Here's how the part is built. I have some questions about the finished solid (model axes, mm). Round coordinates to 2 decimals unless told otherwise and drop trailing zeros. Loops run counter-clockwise (first coordinate to the right, second up) from the corner with the lowest first, then second, coordinate; pieces in that order, holes last. Notation, with made-up numbers: M 9,83.5 L 19,83.5 A17 ccw 19,102.5 Z; hole C -23.5,57 d6. An arc over 180 degrees is marked long. Answer as a JSON object with one key per item and string values.
from build123d import *

# Parameters (mm, degrees)
SKETCH1_W           = 250
SKETCH1_H           = 150
SKETCH1_R           = 1.5
SKETCH1_R_2         = 10
BOSS_EXTRUDE1_DEPTH = 4


with BuildPart() as part:
    # Sketch1 → Boss-Extrude1 (new body)
    with BuildSketch(Plane.XY):
        with Locations((64.901502586, -41.133333333)):
            Rectangle(SKETCH1_W, SKETCH1_H)
        with Locations((-32.098497414, -92.133333333)):
            Circle(SKETCH1_R, mode=Mode.SUBTRACT)
        with Locations((-17.098497414, -92.133333333)):
            Circle(SKETCH1_R, mode=Mode.SUBTRACT)
        with Locations((-32.098497414, -107.133333333)):
            Circle(SKETCH1_R, mode=Mode.SUBTRACT)
        with Locations((-47.098497414, -92.133333333)):
            Circle(SKETCH1_R, mode=Mode.SUBTRACT)
        with Locations((-32.098497414, -77.133333333)):
            Circle(SKETCH1_R, mode=Mode.SUBTRACT)
        with Locations((176.901502586, -92.133333333)):
            Circle(SKETCH1_R, mode=Mode.SUBTRACT)
        with Locations((161.901502586, -92.133333333)):
            Circle(SKETCH1_R, mode=Mode.SUBTRACT)
        with Locations((161.901502586, -77.133333333)):
            Circle(SKETCH1_R, mode=Mode.SUBTRACT)
        with Locations((146.901502586, -92.133333333)):
            Circle(SKETCH1_R, mode=Mode.SUBTRACT)
        with Locations((161.901502586, -107.133333333)):
            Circle(SKETCH1_R, mode=Mode.SUBTRACT)
        with Locations((176.901502586, 9.866666667)):
            Circle(SKETCH1_R, mode=Mode.SUBTRACT)
        with Locations((161.901502586, 9.866666667)):
            Circle(SKETCH1_R, mode=Mode.SUBTRACT)
        with Locations((161.901502586, 24.866666667)):
            Circle(SKETCH1_R, mode=Mode.SUBTRACT)
        with Locations((146.901502586, 9.866666667)):
            Circle(SKETCH1_R, mode=Mode.SUBTRACT)
        with Locations((161.901502586, -5.133333333)):
            Circle(SKETCH1_R, mode=Mode.SUBTRACT)
        with Locations((-17.098497414, 9.866666667)):
            Circle(SKETCH1_R, mode=Mode.SUBTRACT)
        with Locations((-32.098497414, 9.866666667)):
            Circle(SKETCH1_R, mode=Mode.SUBTRACT)
        with Locations((-32.098497414, 24.866666667)):
            Circle(SKETCH1_R, mode=Mode.SUBTRACT)
        with Locations((-47.098497414, 9.866666667)):
            Circle(SKETCH1_R, mode=Mode.SUBTRACT)
        with Locations((-32.098497414, -5.133333333)):
            Circle(SKETCH1_R, mode=Mode.SUBTRACT)
        with Locations((-32.098497414, -41.133333333)):
            Circle(SKETCH1_R, mode=Mode.SUBTRACT)
        with Locations((161.901502586, -41.133333333)):
            Circle(SKETCH1_R, mode=Mode.SUBTRACT)
        with Locations((64.901502586, 9.866666667)):
            Circle(SKETCH1_R, mode=Mode.SUBTRACT)
        with Locations((64.901502586, -92.133333333)):
            Circle(SKETCH1_R, mode=Mode.SUBTRACT)
        with Locations((94.901502586, -41.133333333)):
            Circle(SKETCH1_R_2, mode=Mode.SUBTRACT)
        with Locations((34.901502586, -41.133333333)):
            Circle(SKETCH1_R_2, mode=Mode.SUBTRACT)
    extrude(amount=BOSS_EXTRUDE1_DEPTH)


solid = part.part
Item 1: If I drill on L1, parallel to X at y = 24.5, z = 2.3; L2, parallel to Y at x = 177.5, z = 0.65; L3, parallel to X at y = -76.5, z = 3.3, over which ranges is the centre line in solid material (lowest first)? Write a range as from..to.
Solution:
{"L1": "x = -60.1..-33.55, -30.64..160.45, 163.36..189.9", "L2": "y = -116.13..-93.51, -90.76..8.49, 11.24..33.87", "L3": "x = -60.1..-33.46, -30.74..160.54, 163.26..189.9"}
Item 2: For P1, Ø2.5, axis at x = 161.9, y = -41.13, coming from the +Z side, with a flat end and sliding along its axis, tell me the tip position at first contact or that it passes through.
Solution:
{"P1": "passes through"}
Item 3: We'd pull the mould along Y, two halves only. Please class faces 1 (the face through (24.91, -40.69, 1.97)), 2 (the face through (63, -40, 4)): +Y half, -Y half, draft (parallel to the pull), parting line (faces both ways), or undercut.
Solution:
{"face 1": "undercut", "face 2": "draft"}
Item 4: I want a section at A-A on x = 102.5. List the corners of the cut face in (y, z) for me.
Solution:
{"outline": "M -116.13,0 L -47.63,0 L -47.63,4 L -116.13,4 Z; M -34.63,0 L 33.87,0 L 33.87,4 L -34.63,4 Z"}
Item 5: I want a section at B-B on z = 2. Count the separate pieces of the cut face and the enclosed holes in it, plus the area to 3 significant figures.
Solution:
{"separate pieces": "1", "enclosed holes": "26", "area": "36,700 mm2"}
Item 6: I want a section at C-C on y = -36.5. List the corners of the cut face in (x, z) for me, plus the area to 3 significant figures.
Solution:
{"outline": "M -60.1,0 L 26.04,0 L 26.04,4 L -60.1,4 Z; M 43.76,0 L 86.04,0 L 86.04,4 L 43.76,4 Z; M 103.76,0 L 189.9,0 L 189.9,4 L 103.76,4 Z", "area": "858 mm2"}
